Part model, mm, in its own coordinate system. Face numbers are marked on the shaded views. A direction names the side the tool comes from. Give positions to 0.01 mm unless a question says otherwise; leave off trailing zeros. Order: outer loops, then holes, each group sorted by start corner. A loop starts at its lowest first (then second) coordinate and runs counter-clockwise, first axis right, second up. Notation, with made-up numbers: (49, 28) - (86, 28) arc R15 ccw to (86, 34) - close; hole circle Ø1 at (19, 35). An arc over 180 degrees is marked (long way). Use a Markdown table: item, result. Add a question column.
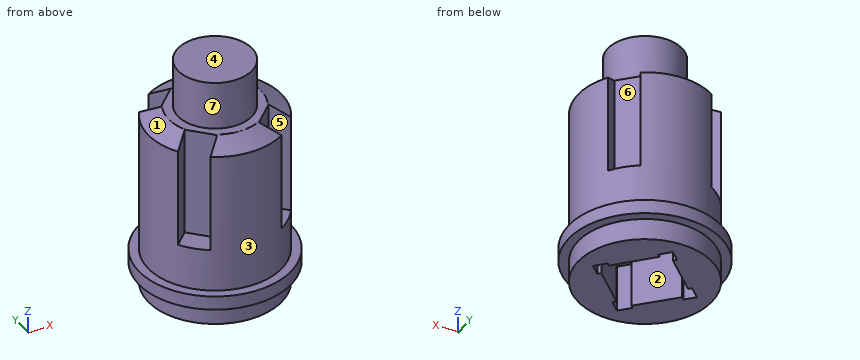
from build123d import *

# Parameters (mm, degrees)
EXTRUDE_1_DEPTH      = 0.3
EXTRUDE_1_DEPTH_BACK = 16.969059
SKETCH_1_R           = 7.2
SKETCH_1_2_R         = 7.2
EXTRUDE_2_DEPTH      = 2
SKETCH_2_R           = 3.99
EXTRUDE_3_DEPTH      = 6.330940566
SKETCH_2_3_R         = 5
SKETCH_2_3_R_2       = 3.99
EXTRUDE_4_DEPTH      = 1.130940566
CHAMFER_1_SIZE       = 2.3
CHAMFER_1_SIZE_2     = 1.121784954
EXTRUDE_START        = 0.3
SKETCH_3_R           = 8.2
SKETCH_3_R_2         = 7.2
EXTRUDE_5_DEPTH      = 1.5
CUT_EXTRUDE_START    = 0.1
SKETCH_5_R           = 31.525677416
CUT_EXTRUDE_1_DEPTH  = 412.780220489
CUT_EXTRUDE_2_DEPTH  = 5
MOVE_FACE_1_BY       = 0.8


with BuildPart() as part:
    # Эскиз1 → Бобышка-Вытянуть1 (new, two sides: drawn at the far end of the back side and taken through both)
    with BuildSketch(Plane.XY.offset(-EXTRUDE_1_DEPTH_BACK)):
        with Locations((-387.828180977, 102.977102389)):
            Circle(SKETCH_1_R)
        Polygon((-387.828180977, 97.956644243), (-382.80772283, 102.977102389), (-387.757470299, 108.068271214), (-392.848639123, 102.977102389), align=None, mode=Mode.SUBTRACT)
    extrude(amount=EXTRUDE_1_DEPTH + EXTRUDE_1_DEPTH_BACK)

    # Эскиз1<2> → Бобышка-Вытянуть2 (add)
    with BuildSketch(Plane.XY):
        with Locations((-387.828180977, 102.977102389)):
            Circle(SKETCH_1_2_R)
    extrude(amount=EXTRUDE_2_DEPTH)

    # Эскиз2 → Бобышка-Вытянуть3 (add)
    with BuildSketch(Plane.XY.offset(2)):
        with Locations((-387.828180977, 102.977102389)):
            Circle(SKETCH_2_R)
    extrude(amount=EXTRUDE_3_DEPTH)

    # Эскиз2<3> → Бобышка-Вытянуть4 (add)
    with BuildSketch(Plane.XY.offset(2)):
        with Locations(Location((-387.828180977, 102.977102389, 0), (0, 0, 180))):
            Circle(SKETCH_2_3_R)
        with Locations((-387.828180977, 102.977102389)):
            Circle(SKETCH_2_3_R_2, mode=Mode.SUBTRACT)
    extrude(amount=EXTRUDE_4_DEPTH)

    # Фаска1
    # the kernel refuses this chamfer: 2.3, 1.121784954 mm, written as the material it adds along each edge
    with BuildSketch(Plane(origin=(-387.828180977, 102.977102389, 2), x_dir=(-1, 0, 0), z_dir=(0, 1, 0))) as chamfer_1_piece_1_section:
        Polygon((5 + CHAMFER_1_SIZE, 0), (5, CHAMFER_1_SIZE_2), (5, 0), align=None)
    chamfer_1_piece_1 = revolve(axis=Axis((-387.828180977, 102.977102389, 2), (0, 0, 1)), mode=Mode.PRIVATE)
    chamfer_1_piece_1 = chamfer_1_piece_1 & Plane(origin=(-387.828180977, 102.977102389, 2.571661691), x_dir=(1, 0, 0), z_dir=(0, 0, -1)) * Cylinder(7.2, 30, mode=Mode.PRIVATE)
    add(chamfer_1_piece_1)

    # Эскиз3 → Бобышка-Вытянуть5 (add)
    with BuildSketch(Plane.XY.offset(-14.969059434).offset(EXTRUDE_START)):
        with Locations((-387.828180977, 102.977102389)):
            Circle(SKETCH_3_R)
        with Locations(Location((-387.828180977, 102.977102389, 0), (0, 0, 180))):
            Circle(SKETCH_3_R_2, mode=Mode.SUBTRACT)
    extrude(amount=EXTRUDE_5_DEPTH)

    # Эскиз5 → Вырез-Вытянуть1 (cut, through all)
    with BuildSketch(Plane(origin=(0, 0, -8.460000998), x_dir=(-1, 0, 0), z_dir=(0, 0, -1)).offset(CUT_EXTRUDE_START)):
        with Locations((387.828180977, 102.977102389)):
            Circle(SKETCH_5_R)
        with BuildLine():
            Line((385.524514896, 98.471917351), (383.813441597, 96.760844053))
            ThreePointArc((383.813441597, 96.760844053), (387.783841084, 95.57723523), (391.7681393, 96.713179624))
            Line((391.7681393, 96.713179624), (390.070624315, 98.410694608))
            Line((390.070624315, 98.410694608), (392.333366015, 100.673436308))
            Line((392.333366015, 100.673436308), (394.044439314, 98.962363009))
            ThreePointArc((394.044439314, 98.962363009), (395.228048136, 102.932762497), (394.092103743, 106.917060712))
            Line((394.092103743, 106.917060712), (392.394588758, 105.219545727))
            Line((392.394588758, 105.219545727), (390.131847058, 107.482287427))
            Line((390.131847058, 107.482287427), (391.842920357, 109.193360726))
            ThreePointArc((391.842920357, 109.193360726), (387.87252087, 110.376969549), (383.888222654, 109.241025155))
            Line((383.888222654, 109.241025155), (385.585737639, 107.54351017))
            Line((385.585737639, 107.54351017), (383.322995939, 105.280768471))
            Line((383.322995939, 105.280768471), (381.61192264, 106.99184177))
            ThreePointArc((381.61192264, 106.99184177), (380.428313818, 103.021442282), (381.564258211, 99.037144067))
            Line((381.564258211, 99.037144067), (383.261773196, 100.734659051))
            Line((383.261773196, 100.734659051), (385.524514896, 98.471917351))
        make_face(mode=Mode.SUBTRACT)
    extrude(amount=-CUT_EXTRUDE_1_DEPTH, mode=Mode.SUBTRACT)

    # Эскиз6 → Вырез-Вытянуть2 (cut)
    with BuildSketch(Plane(origin=(0, 0, -16.969059434), x_dir=(-1, 0, 0), z_dir=(0, 0, -1))):
        Polygon((392.467199832, 102.029977673), (391.330034344, 103.13555523), (392.279390791, 104.112036147), (393.414324548, 102.977102389), align=None)
        Polygon((383.255874897, 104.011882353), (384.259667783, 103.035972602), (383.236040731, 101.983099063), (382.245993053, 102.973146742), align=None)
        Polygon((386.771925298, 98.447214497), (387.844642377, 99.550580636), (388.931315265, 98.494093106), (387.828180977, 97.390958818), align=None)
        Polygon((387.753458546, 108.637968392), (386.741266863, 107.596856947), (387.74505975, 106.620947196), (388.743506224, 107.647920713), align=None)
    extrude(amount=-CUT_EXTRUDE_2_DEPTH, mode=Mode.SUBTRACT)

    # Move Face 1: a face moved inward by 0.8
    extrude(part.faces().sort_by_distance((-387.816313451, 103.000672615, 0))[0], amount=MOVE_FACE_1_BY, dir=(0, 0, 1), mode=Mode.SUBTRACT)


solid = part.part
1. Mould opens along Y. For the marked faces 4, 5, 6 and 7 say: released by +Y, released by -Y, zero draft, split by the parting line, or undercut.
2. Cut at B-B (z = -9.5). Write the cut outline in (x, y), plus the area to 3 significant figures.
3. Cut at A-A (z = 0.25). Write the cut outline in (x, y).
4. Pin check, flat tips, straight feed: P1, Ø1, axis at x = -385, z = -14.5, coming from the +Y side; P2, Ø0.7, axis at x = -387.5, y = 107.5, coming from the -Z side; P3, Ø1.5, axis at y = 99, z = -3, coming from the +X side. Stop position of each tip, or through.
5. Tool access for the marked faces 1, 2 and 3: list every direction of +Z, -Z, +X, -X, +Y, -Y with a clear straight run to the whole face (end or side of a thin tool).
6. Drill centre lines: probe 1 along Y at (x, z) = (-391.5, -1); probe 2 along Z at (x, y) = (-380.75, 100.5); probe 3 along Y at (x, z) = (-386.5, -15.5). Where is each one in solid material? Low to high. Write a range as [from, to].
Responses:
| question | item | result |
|---|---|---|
| 1 | face 4 | zero draft |
| 1 | face 5 | released by -Y |
| 1 | face 6 | undercut |
| 1 | face 7 | split by the parting line |
| 2 | outline | circle Ø14.4 at (-387.83, 102.98); hole (-392.85, 102.98) - (-387.83, 97.96) - (-382.81, 102.98) - (-387.76, 108.07) - close |
| 2 | area | 112 mm² |
| 3 | outline | (-393.95, 106.77) arc R7.2 ccw to (-393.9, 99.11) - (-392.33, 100.67) - (-390.07, 98.41) - (-391.62, 96.86) arc R7.2 ccw to (-383.96, 96.91) - (-385.52, 98.47) - (-383.26, 100.73) - (-381.71, 99.18) arc R7.2 ccw to (-381.76, 106.85) - (-383.32, 105.28) - (-385.59, 107.54) - (-384.03, 109.1) arc R7.2 ccw to (-391.7, 109.05) - (-390.13, 107.48) - (-392.39, 105.22) - close; hole (-392.85, 102.98) - (-387.83, 97.96) - (-382.81, 102.98) - (-387.76, 108.07) - close |
| 4 | P1 | stops at y = 110.84 |
| 4 | P2 | stops at z = -11.97 |
| 4 | P3 | stops at x = -381.39 |
| 5 | face 1 | +Z, -X |
| 5 | face 2 | -Z |
| 5 | face 3 | +Z |
| 6 | probe 1 | y = [96.78, 96.98], [99.84, 101.63], [104.33, 106.11], [108.85, 109.17] |
| 6 | probe 2 | z = [-14.67, -13.17] |
| 6 | probe 3 | y = [95.9, 99.28], [106.77, 110.05] |
